from build123d import *

# Parameters (mm, degrees)
F0_W     = 38
F0_H     = 40
F0_W_2   = 33.907328
F0_H_2   = 36
F1_DEPTH = 20
F2_W     = 42
F2_H     = 44
F3_DEPTH = 2


with BuildPart() as f1:
    # F0 (on Front) → F1 (new body)
    with BuildSketch(Plane.XZ):
        with Locations((1.039558, -20.108323)):
            Rectangle(F0_W, F0_H)
        with Locations((0.993222, -20.108323)):
            Rectangle(F0_W_2, F0_H_2, mode=Mode.SUBTRACT)
    extrude(amount=F1_DEPTH)

    # F2 (on Front) → F3 (join)
    with BuildSketch(Plane.XZ):
        with Locations((1.039558, -20.108323)):
            Rectangle(F2_W, F2_H)
    extrude(amount=-F3_DEPTH)


solid = f1.part
The model under review builds one solid part; all positions refer to its coordinate system, in mm. A direction names the side the tool comes from. Coordinates: 2 decimals unless noted, no trailing zeros. Write each loop counter-clockwise with the first axis right and the second up, starting at its lowest first coordinate (ties: lowest second). Pieces come first, ordered by that corner, then holes. Notation, with made-up numbers: (25, 15.5) - (76, 15.5) arc R26 ccw to (76, 38.5) - close; hole circle Ø3 at (39, -12). An arc over 180 degrees is marked (long way). Answer as a JSON object with one key per item and string values. Group by question number.
1. To check wall thickness, follow probe 1 along Z at (x, y) = (10, -1.5); probe 2 along X at (y, z) = (-10.5, -11); probe 3 along Y at (x, z) = (-3.5, -5). State the ranges of each line that lie inside material, in increasing order.
2. Add section A-A (y = -12). Give the boundary of the cut face in (x, z).
3. Add section B-B (z = -17.5). Give the boundary of the cut face in (x, y).
4. Mouldability with a two-part tool opening along X and no side actions: class faces 1 (the face through (22.04, 1, -20)), 2 (the face through (1, -10, -38.108)), 3 (the face through (1, 0, -20)), 4 (the face through (1, 1, 1.892)) as pulls with the +X half, pulls with the -X half, needs draft (parallel to the pull), parting line crosses it, or undercut.
5. Clearance check with flat-ended pins moving along their axes: pin 1 Ø10 at (x, y) = (-4, -10) entering from +Z; pin 2 Ø6 at (y, z) = (-14.5, -12) entering from -X; pin 3 Ø3 at (x, z) = (11, -35) entering from -Y. State where each tip first meets the part, or that it passes through.
6. Machinability: for faces 5 (the face through (-17.96, -10, -20)), 6 (the face through (20.04, -10, -20)), 7 (the face through (17.947, -10, -20)), 8 (the face through (1, -10, -40.108)), 9 (the face through (1, -10, -0.108)), which of the approach directions +Z, -Z, +X, -X, +Y, -Y give a long, thin tool a straight path to every point of the face, cutting with its end or side? Answer none if there is none.
7. Add section D-D (x = 9). Give the boundary of the cut face in (y, z).
8. Add section C-C (x = -17). Give the boundary of the cut face in (y, z), plus the area to 3 significant figures.
Findings:
{
 "1": {"probe 1": "-40.11 to -38.11, -2.11 to -0.11", "probe 2": "-17.96 to -15.96, 17.95 to 20.04", "probe 3": "0 to 2"},
 "2": {"outline": "(-17.96, -40.11) - (20.04, -40.11) - (20.04, -0.11) - (-17.96, -0.11) - close; hole (-15.96, -38.11) - (17.95, -38.11) - (17.95, -2.11) - (-15.96, -2.11) - close"},
 "3": {"outline": "(-19.96, 0) - (-17.96, 0) - (-17.96, -20) - (-15.96, -20) - (-15.96, 0) - (17.95, 0) - (17.95, -20) - (20.04, -20) - (20.04, 0) - (22.04, 0) - (22.04, 2) - (-19.96, 2) - close"},
 "4": {"face 1": "pulls with the +X half", "face 2": "undercut", "face 3": "undercut", "face 4": "needs draft"},
 "5": {"pin 1": "z = -0.11", "pin 2": "x = -17.96", "pin 3": "y = 0"},
 "6": {"face 5": "+Z, -Z, -X, -Y", "face 6": "+Z, -Z, +X, -Y", "face 7": "-Y", "face 8": "-Z, +X, -X, -Y", "face 9": "+Z, +X, -X, -Y"},
 "7": {"outline": "(-20, -40.11) - (0, -40.11) - (0, -42.11) - (2, -42.11) - (2, 1.89) - (0, 1.89) - (0, -0.11) - (-20, -0.11) - (-20, -2.11) - (0, -2.11) - (0, -38.11) - (-20, -38.11) - close"},
 "8": {"outline": "(-20, -40.11) - (0, -40.11) - (0, -42.11) - (2, -42.11) - (2, 1.89) - (0, 1.89) - (0, -0.11) - (-20, -0.11) - close", "area": "888 mm²"}
}
